For this review, use the dimensioned drawing (mm, ordinates from the lowest corner) and the shaded views. A direction names the side the tool comes from. Coordinates: 2 decimals unless noted, no trailing zeros. Loops run counter-clockwise (first coordinate to the right, second up) from the corner with the lowest first, then second, coordinate; pieces in that order, holes last.
1. Clearance check with flat-ended pins moving along their axes: P1, Ø10, axis at x = 35.5, y = 20.5, coming from the -Z side; P2, Ø1.5, axis at x = 45.5, z = 8.5, coming from the -Y side; P3, Ø8, axis at x = 24.5, z = 39, coming from the -Y side; P4, Ø4.5, axis at x = 50.4, y = 40.4, coming from the +Z side. State where each tip first meets the part, or that it passes through.
2. Machinability: for the marked faces 1, 2 and 3, which of the approach directions +Z, -Z, +X, -X, +Y, -Y give a long, thin tool a straight path to every point of the face, cutting with its end or side? Answer none if there is none.
3. Take a section at D-D, the plane z = 42. State the section outline as (x, y) points, then the cut area to 3 significant figures.
4. Take a section at B-B, the plane y = 22.7. State the section outline as (x, z) points.
5. To check wall thickness, follow probe 1 along Y at (x, z) = (50.4, 7.3); probe 2 along Z at (x, y) = (51, 34.5); probe 3 along Z at (x, y) = (2, 16.5). State the ranges of each line that lie inside material, in increasing order.
6. Take a section at C-C, the plane z = 3. State the section outline as (x, y) points, then the cut area to 3 significant figures.
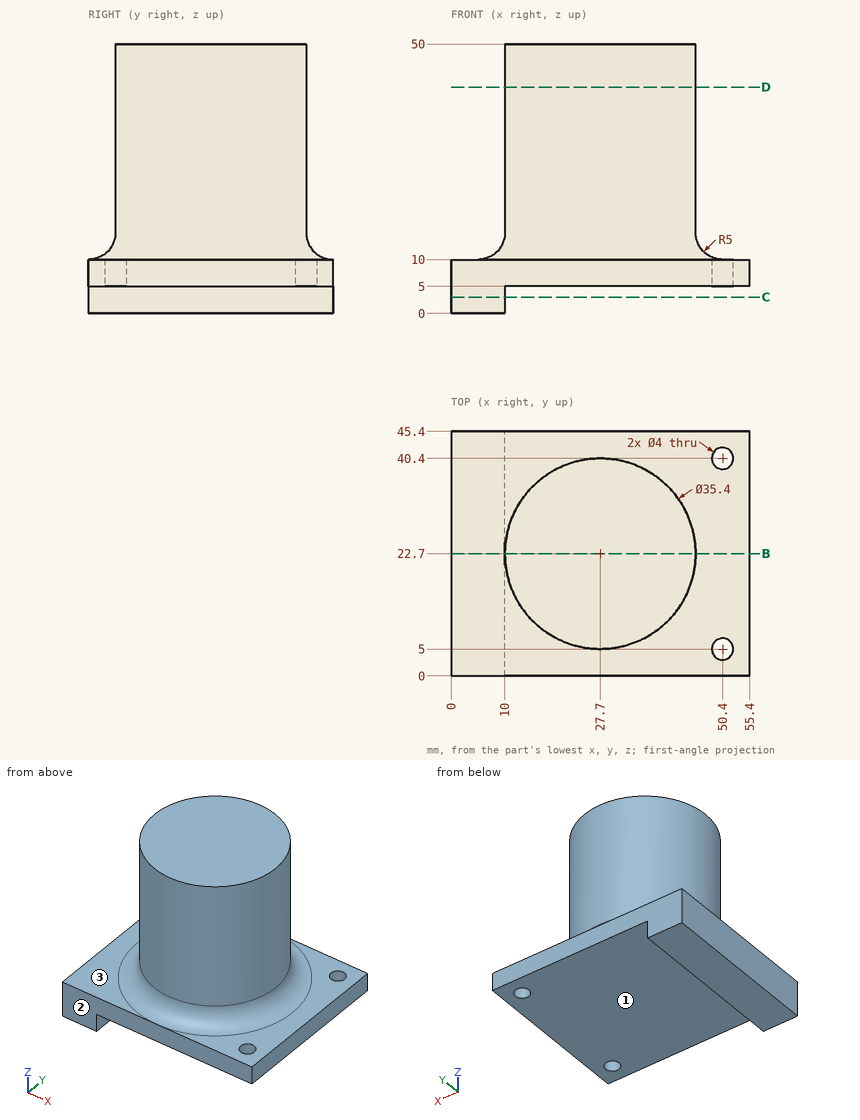
Results list:
1. P1: stops at z = 5
1. P2: stops at y = 0
1. P3: stops at y = 5
1. P4: stops at z = 10
2. face 1: -Z, +X, +Y, -Y
2. face 2: +Z, -Z, +X, -X, -Y
2. face 3: +Z
3. outline: circle Ø35.4 at (27.7, 22.7)
3. area: 984 mm2
4. outline: (0, 0) - (10, 0) - (10, 5) - (55.4, 5) - (55.4, 10) - (50.4, 10) arc R5 cw to (45.4, 15) - (45.4, 50) - (10, 50) - (10, 15) arc R5 cw to (5, 10) - (0, 10) - close
5. probe 1: y = 0 to 3, 7 to 38.4, 42.4 to 45.4
5. probe 2: z = 5 to 10
5. probe 3: z = 0 to 10
6. outline: (0, 0) - (10, 0) - (10, 45.4) - (0, 45.4) - close
6. area: 454 mm2
